Could you check a few things on this model? Use its own coordinates, in mm. A direction names the side the tool comes from. Round coordinates to 2 decimals unless told otherwise and drop trailing zeros. Order: outer loops, then holes, each group sorted by start corner. A loop starts at its lowest first (then second) coordinate and runs counter-clockwise, first axis right, second up. Notation, with made-up numbers: (62, -26.75) -> (108, -26.75) arc R16 ccw to (108, -6.75) -> close; hole circle Ø11 at (63.5, 26.25). An arc over 180 degrees is marked (long way). One line per question, with ' | ' between items.
```python
from build123d import *

# Parameters (mm, degrees)
F0_W     = 40
F0_H     = 27
F0_R     = 7.5
F1_DEPTH = 10
F2_DEPTH = 2
F3_R     = 2


with BuildPart() as f1:
    # F0 (on Top) → F1 (new body)
    with BuildSketch(Plane.XY):
        Rectangle(F0_W, F0_H)
        Circle(F0_R, mode=Mode.SUBTRACT)
        Circle(F0_R)
    extrude(amount=F1_DEPTH)

    # F0 (on Top) → F2 (cut)
    with BuildSketch(Plane.XY):
        Circle(F0_R)
    extrude(amount=F2_DEPTH, mode=Mode.SUBTRACT)

    # F3
    f3_edges = [f1.edges().sort_by_distance(p)[0] for p in [
        (20, -13.5, 5),
        (20, 13.5, 5),
        (-20, 13.5, 5),
        (-20, -13.5, 5),
    ]]
    fillet(f3_edges, radius=F3_R)


solid = f1.part
```
1. I need wall thicknesses on probe 1 along Y at (x, z) = (0, 1.4); probe 2 along Z at (x, y) = (-4, 1.25); probe 3 along Y at (x, z) = (18.5, 4). Which ranges of each line are inside material? Lowest first, please.
From the geometry:
probe 1: y = -13.5 to -7.5, 7.5 to 13.5 | probe 2: z = 2 to 10 | probe 3: y = -13.44 to 13.44
2. If we mould it in two halves opening along Y, with no side actions, what happens to faces 1 (the face through (19.4, 12.93, 5.07)), 2 (the face through (-7.493, 0.33, 0.986)), 3 (the face through (0, 0, 10)), 4 (the face through (0, -13.5, 5))? For each: pulls with the +Y half, pulls with the -Y half, needs draft (parallel to the pull), parting line crosses it, or undercut.
From the geometry:
face 1: pulls with the +Y half | face 2: undercut | face 3: needs draft | face 4: pulls with the -Y half
3. I want a section at C-C on y = 0. List the corners of the cut face in (x, z) for me.
From the geometry:
outline: (-20, 0) -> (-7.5, 0) -> (-7.5, 2) -> (7.5, 2) -> (7.5, 0) -> (20, 0) -> (20, 10) -> (-20, 10) -> close
4. I'm going to push a flat-ended pin straight in: pin 1 (1 mm diameter, centred on x = -5.5, y = -2.5, fed in from -Z). Where does the tip first touch, or does it pass through?
From the geometry:
pin 1: stops at z = 2
5. I want a section at A-A on z = 1.5. List the corners of the cut face in (x, y) for me, and give its area (3 significant figures).
From the geometry:
outline: (-20, -11.5) arc R2 ccw to (-18, -13.5) -> (18, -13.5) arc R2 ccw to (20, -11.5) -> (20, 11.5) arc R2 ccw to (18, 13.5) -> (-18, 13.5) arc R2 ccw to (-20, 11.5) -> close; hole circle Ø15 at (0, 0) | area: 900 mm²
6. I want a section at B-B on x = 0. List the corners of the cut face in (y, z) for me, and give its area (3 significant figures).
From the geometry:
outline: (-13.5, 0) -> (-7.5, 0) -> (-7.5, 2) -> (7.5, 2) -> (7.5, 0) -> (13.5, 0) -> (13.5, 10) -> (-13.5, 10) -> close | area: 240 mm²
7. On a 3-axis mill with a long thin cutter (end or side, diameter ignored), from which of +Z, -Z, +X, -X, +Y, -Y can I reach the whole of each face in a straight line? I mean faces 5 (the face through (-19.43, -12.9, 5.07)), 6 (the face through (0, 0, 2)). Say none if no direction works.
From the geometry:
face 5: +Z, -Z, -X, -Y | face 6: -Z
